For this review, use the dimensioned drawing (mm, ordinates from the lowest corner) and the shaded views. A direction names the side the tool comes from. Coordinates: 2 decimals unless noted, no trailing zeros. Write each loop counter-clockwise with the first axis right and the second up, starting at its lowest first coordinate (ties: lowest second). Pieces come first, ordered by that corner, then holes.
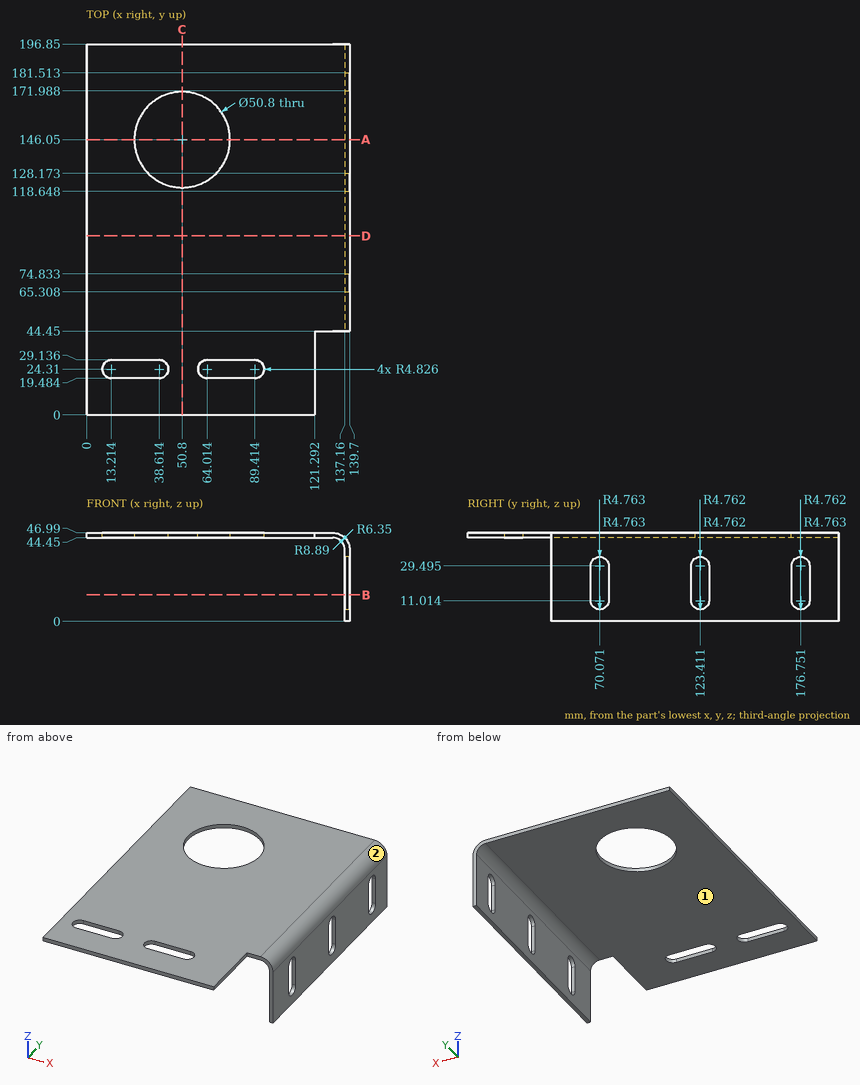
(1) Insertion check: pin 1 Ø9 at (x, z) = (133, 17) entering from -Y; pin 2 Ø3 at (y, z) = (27, 46) entering from +X; pin 3 Ø3 at (x, y) = (34.5, 128.5) entering from -Z. Each pin has a flat end and moves straight along its axis. Give the tip position at first contact, or say it passes through.
(2) Consider section B-B (z = 14). Give the boundary of the cut face in (x, y).
(3) Consider section D-D (y = 95). Give the boundary of the cut face in (x, z).
(4) Consider section A-A (y = 146.05). Give the boundary of the cut face in (x, z).
(5) Consider section C-C (x = 50.8). Give the boundary of the cut face in (y, z).
(6) For the marked faces 1 and 2, list the 3-axis set-ups (+Z, -Z, +X, -X, +Y, -Y) from which the entire face can be reached by the end or side of a thin tool; tool diameter is ignored.
(7) Wall thickness on line 1 (Y direction, x = 50, z = 45); line 2 (Z direction, x = 25, y = 165); line 3 (X direction, y = 148, z = 19): over which ranges is each line inside the solid? List them lowest first.
Results:
1. pin 1: stops at y = 44.45
1. pin 2: stops at x = 121.29
1. pin 3: stops at z = 44.45
2. outline: (137.16, 44.45) - (139.7, 44.45) - (139.7, 65.31) - (137.16, 65.31) - close; (137.16, 74.83) - (139.7, 74.83) - (139.7, 118.65) - (137.16, 118.65) - close; (137.16, 128.17) - (139.7, 128.17) - (139.7, 171.99) - (137.16, 171.99) - close; (137.16, 181.51) - (139.7, 181.51) - (139.7, 196.85) - (137.16, 196.85) - close
3. outline: (0, 44.45) - (130.81, 44.45) arc R6.35 cw to (137.16, 38.1) - (137.16, 0) - (139.7, 0) - (139.7, 38.1) arc R8.89 ccw to (130.81, 46.99) - (0, 46.99) - close
4. outline: (0, 44.45) - (25.4, 44.45) - (25.4, 46.99) - (0, 46.99) - close; (76.2, 44.45) - (130.81, 44.45) arc R6.35 cw to (137.16, 38.1) - (137.16, 0) - (139.7, 0) - (139.7, 38.1) arc R8.89 ccw to (130.81, 46.99) - (76.2, 46.99) - close
5. outline: (0, 44.45) - (120.65, 44.45) - (120.65, 46.99) - (0, 46.99) - close; (171.45, 44.45) - (196.85, 44.45) - (196.85, 46.99) - (171.45, 46.99) - close
6. face 1: -Z, -X, +Y, -Y
6. face 2: +Z, +X, +Y, -Y
7. line 1: y = 0 to 120.66, 171.44 to 196.85
7. line 2: z = 44.45 to 46.99
7. line 3: x = 137.16 to 139.7
